```python
from build123d import *

# Parameters (mm, degrees)
F0_R          = 2.75
F0_R_2        = 13
F1_DEPTH      = 10
F1_DEPTH_BACK = 10
F2_R          = 13
F2_R_2        = 5
F3_DEPTH      = 4
F3_DEPTH_BACK = 4
F4_R          = 3.25
F5_DEPTH      = 32.501
F6_R          = 5.4
F7_DEPTH      = 1.5


with BuildPart() as f1:
    # F0 (on Front) → F1 (new body, two sides)
    with BuildSketch(Plane.XZ) as f1_sk:
        Polygon((-30, -16.25), (30, -16.25), (30, 16.25), (17, 16.25), (17, 26.75), (-17, 26.75), (-17, 16.25), (-30, 16.25), align=None)
        with Locations((-23, -9.25)):
            Circle(F0_R, mode=Mode.SUBTRACT)
        with Locations((23, -9.25)):
            Circle(F0_R, mode=Mode.SUBTRACT)
        with Locations((-23, 8.75)):
            Circle(F0_R, mode=Mode.SUBTRACT)
        with Locations((0, 8.75)):
            Circle(F0_R_2, mode=Mode.SUBTRACT)
        with Locations((23, 8.75)):
            Circle(F0_R, mode=Mode.SUBTRACT)
    extrude(amount=F1_DEPTH)
    extrude(f1_sk.sketch, amount=-F1_DEPTH_BACK)

    # F2 (on Front) → F3 (join, two sides)
    with BuildSketch(Plane.XZ) as f3_sk:
        with Locations((0, 8.75)):
            Circle(F2_R)
        with Locations((0, 8.75)):
            Circle(F2_R_2, mode=Mode.SUBTRACT)
    extrude(amount=F3_DEPTH)
    extrude(f3_sk.sketch, amount=-F3_DEPTH_BACK)

    # F4 (on face) → F5 (cut, through all)
    with BuildSketch(Plane.XY.offset(16.25)):
        with Locations((-23, 0)):
            Circle(F4_R)
        with Locations((23, 0)):
            Circle(F4_R)
    extrude(amount=-F5_DEPTH, mode=Mode.SUBTRACT)

    # F6 (on face) → F7 (cut)
    with BuildSketch(Plane.XY.offset(16.25)):
        with Locations((-23, 0)):
            Circle(F6_R)
        with Locations((23, 0)):
            Circle(F6_R)
    extrude(amount=-F7_DEPTH, mode=Mode.SUBTRACT)


solid = f1.part
```
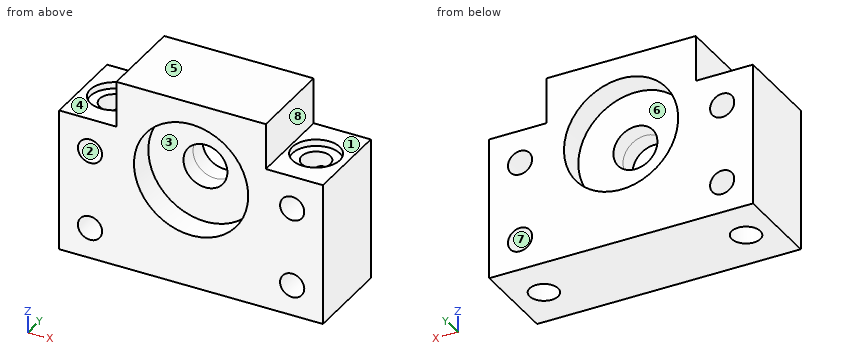
Check sheet for the modelled part. Datum: model origin and axes. Units: mm. Face numbers are marked on the shaded views. A direction names the side the tool comes from. Round coordinates to 2 decimals unless told otherwise and drop trailing zeros. Loops run counter-clockwise (first coordinate to the right, second up) from the corner with the lowest first, then second, coordinate; pieces in that order, holes last. Notation, with made-up numbers: (-7, -9.75) -> (-1, -9.75) arc R16 ccw to (-1, 7.25) -> close; hole circle Ø4 at (76.25, -37). An arc over 180 degrees is marked (long way). Answer in a Markdown table with one row per item.
Q1. Sectioned sample at D-D on x = 0. Enter the section's corners in (y, z).
Data:
| item | result |
|---|---|
| outline | (-10, -16.25) -> (10, -16.25) -> (10, -4.25) -> (4, -4.25) -> (4, 3.75) -> (-4, 3.75) -> (-4, -4.25) -> (-10, -4.25) -> close; (-10, 21.75) -> (-4, 21.75) -> (-4, 13.75) -> (4, 13.75) -> (4, 21.75) -> (10, 21.75) -> (10, 26.75) -> (-10, 26.75) -> close |
Q2. Go/stop test with flat-tipped pins: P1, Ø12, axis at x = 21, y = 1.5, coming from the +Z side; P2, Ø1.5, axis at x = 23.5, y = -3.5, coming from the +Z side; P3, Ø10.5, axis at x = -25, y = -0.5, coming from the +Z side; P4, Ø8, axis at x = -1, z = 10, coming from the -Y side. Record where each tip stops, or that it passes through.
Data:
| item | result |
|---|---|
| P1 | stops at z = 26.75 |
| P2 | stops at z = 14.75 |
| P3 | stops at z = 16.25 |
| P4 | stops at y = -4 |
Q3. Release check for a two-part mould opening along X. For the marked faces 5, 6, 7 and 8 record: released by +X, released by -X, zero draft, split by the parting line, or undercut.
Data:
| item | result |
|---|---|
| face 5 | zero draft |
| face 6 | undercut |
| face 7 | undercut |
| face 8 | released by +X |
Q4. Sectioned sample at A-A on z = -9.25. Enter the section's corners in (x, y).
Data:
| item | result |
|---|---|
| outline | (-30, -10) -> (-25.75, -10) -> (-25.75, -1.73) arc R3.25 cw to (-25.75, 1.73) -> (-25.75, 10) -> (-30, 10) -> close; (-20.25, -10) -> (20.25, -10) -> (20.25, -1.73) arc R3.25 cw to (20.25, 1.73) -> (20.25, 10) -> (-20.25, 10) -> (-20.25, 1.73) arc R3.25 cw to (-20.25, -1.73) -> close; (25.75, -10) -> (30, -10) -> (30, 10) -> (25.75, 10) -> (25.75, 1.73) arc R3.25 cw to (25.75, -1.73) -> close |
Q5. Sectioned sample at B-B on x = 23. Enter the section's corners in (y, z), then the cut area to 3 significant figures.
Data:
| item | result |
|---|---|
| outline | (-10, -16.25) -> (-3.25, -16.25) -> (-3.25, -12) -> (-10, -12) -> close; (-10, -6.5) -> (-3.25, -6.5) -> (-3.25, 6) -> (-10, 6) -> close; (-10, 11.5) -> (-3.25, 11.5) -> (-3.25, 14.75) -> (-5.4, 14.75) -> (-5.4, 16.25) -> (-10, 16.25) -> close; (3.25, -16.25) -> (10, -16.25) -> (10, -12) -> (3.25, -12) -> close; (3.25, -6.5) -> (10, -6.5) -> (10, 6) -> (3.25, 6) -> close; (3.25, 11.5) -> (10, 11.5) -> (10, 16.25) -> (5.4, 16.25) -> (5.4, 14.75) -> (3.25, 14.75) -> close |
| area | 284 mm^2 |
Q6. Sectioned sample at C-C on z = 8.75. Give the number of separate pieces and of enclosed holes in the cut face, then the cut area to 3 significant figures.
Data:
| item | result |
|---|---|
| separate pieces | 4 |
| enclosed holes | 0 |
| area | 583 mm^2 |
Q7. Set-up check for the marked faces 1, 2, 3 and 4: record each of +Z, -Z, +X, -X, +Y, -Y from which the full face is reachable in a straight line by a thin tool's end or side.
Data:
| item | result |
|---|---|
| face 1 | +Z, +X, +Y, -Y |
| face 2 | +Y, -Y |
| face 3 | -Y |
| face 4 | +Z, -X, +Y, -Y |
Q8. Thickness scan on L1, parallel to X at y = -6.5, z = -9.25; L2, parallel to Z at x = 23, y = -7; L3, parallel to Y at x = 23, z = -6. Record the ranges inside material, lowest first.
Data:
| item | result |
|---|---|
| L1 | x = -30 to -25.75, -20.25 to 20.25, 25.75 to 30 |
| L2 | z = -16.25 to -12, -6.5 to 6, 11.5 to 16.25 |
| L3 | y = -10 to -3.25, 3.25 to 10 |
